from build123d import *

# Parameters (mm, degrees)
F0_R     = 2
F0_W     = 2.6
F0_H     = 107.6
F0_W_2   = 1.2
F0_H_2   = 1.2
F1_DEPTH = 1
F2_DEPTH = 10


with BuildPart() as f1:
    # F0 (on Top) → F1 (new body)
    with BuildSketch(Plane.XY):
        with BuildLine():
            ThreePointArc((65, 39.2), (57.4433549546, 57.4433549546), (39.2, 65))
            Line((39.2, 65), (-39.2, 65))
            ThreePointArc((-39.2, 65), (-57.4433549546, 57.4433549546), (-65, 39.2))
            Line((-65, 39.2), (-65, -39.2))
            ThreePointArc((-65, -39.2), (-57.4433549546, -57.4433549546), (-39.2, -65))
            Line((-39.2, -65), (39.2, -65))
            ThreePointArc((39.2, -65), (57.4433549546, -57.4433549546), (65, -39.2))
            Line((65, -39.2), (65, 39.2))
        make_face()
        with BuildLine():
            ThreePointArc((-58, -46.1086357947), (-61.4142135624, -47.5228493571), (-60, -44.1086357947))
            ThreePointArc((-60, -44.1086357947), (-58.5857864376, -44.6944222324), (-58, -46.1086357947))
        make_face(mode=Mode.SUBTRACT)
        with BuildLine():
            ThreePointArc((62, -46.1086357947), (58.5857864376, -47.5228493571), (60, -44.1086357947))
            ThreePointArc((60, -44.1086357947), (61.4142135624, -44.6944222324), (62, -46.1086357947))
        make_face(mode=Mode.SUBTRACT)
        with BuildLine():
            ThreePointArc((-58, 32.2913642053), (-58.5857864376, 30.8771506429), (-60, 30.2913642053))
            ThreePointArc((-60, 30.2913642053), (-61.4142135624, 33.7055777676), (-58, 32.2913642053))
        make_face(mode=Mode.SUBTRACT)
        with Locations((-39.2, 60)):
            Circle(F0_R, mode=Mode.SUBTRACT)
        with BuildLine():
            ThreePointArc((-55, 39.2), (-50.3722871427, 50.3722871427), (-39.2, 55))
            Line((-39.2, 55), (-2.5, 55))
            Line((-2.5, 55), (-1.3, 55))
            Line((-1.3, 55), (1.3, 55))
            Line((1.3, 55), (2.5, 55))
            Line((2.5, 55), (39.2, 55))
            ThreePointArc((39.2, 55), (50.3722871427, 50.3722871427), (55, 39.2))
            Line((55, 39.2), (55, -39.2))
            ThreePointArc((55, -39.2), (50.3722871427, -50.3722871427), (39.2, -55))
            Line((39.2, -55), (2.5, -55))
            Line((2.5, -55), (1.3, -55))
            Line((1.3, -55), (-1.3, -55))
            Line((-1.3, -55), (-2.5, -55))
            Line((-2.5, -55), (-39.2, -55))
            ThreePointArc((-39.2, -55), (-50.3722871427, -50.3722871427), (-55, -39.2))
            Line((-55, -39.2), (-55, 39.2))
        make_face(mode=Mode.SUBTRACT)
        with BuildLine():
            ThreePointArc((62, 32.2913642053), (61.4142135624, 30.8771506429), (60, 30.2913642053))
            ThreePointArc((60, 30.2913642053), (58.5857864376, 33.7055777676), (62, 32.2913642053))
        make_face(mode=Mode.SUBTRACT)
        with BuildLine():
            ThreePointArc((41.2, 60), (39.2, 58), (37.2, 60))
            ThreePointArc((37.2, 60), (39.2, 62), (41.2, 60))
        make_face(mode=Mode.SUBTRACT)
        Rectangle(F0_W, F0_H)
        with BuildLine():
            Line((-2.5, 55), (-39.2, 55))
            ThreePointArc((-39.2, 55), (-50.3722871427, 50.3722871427), (-55, 39.2))
            Line((-55, 39.2), (-55, -39.2))
            ThreePointArc((-55, -39.2), (-50.3722871427, -50.3722871427), (-39.2, -55))
            Line((-39.2, -55), (-2.5, -55))
            Line((-2.5, -55), (-2.5, -53.8))
            Line((-2.5, -53.8), (-38.8, -53.8))
            ThreePointArc((-38.8, -53.8), (-49.4066017178, -49.4066017178), (-53.8, -38.8))
            Line((-53.8, -38.8), (-53.8, 38.8))
            ThreePointArc((-53.8, 38.8), (-49.4066017178, 49.4066017178), (-38.8, 53.8))
            Line((-38.8, 53.8), (-2.5, 53.8))
            Line((-2.5, 53.8), (-2.5, 55))
        make_face()
        with BuildLine():
            Line((39.2, 55), (2.5, 55))
            Line((2.5, 55), (2.5, 53.8))
            Line((2.5, 53.8), (38.8, 53.8))
            ThreePointArc((38.8, 53.8), (49.4066017178, 49.4066017178), (53.8, 38.8))
            Line((53.8, 38.8), (53.8, -38.8))
            ThreePointArc((53.8, -38.8), (49.4066017178, -49.4066017178), (38.8, -53.8))
            Line((38.8, -53.8), (2.5, -53.8))
            Line((2.5, -53.8), (2.5, -55))
            Line((2.5, -55), (39.2, -55))
            ThreePointArc((39.2, -55), (50.3722871427, -50.3722871427), (55, -39.2))
            Line((55, -39.2), (55, 39.2))
            ThreePointArc((55, 39.2), (50.3722871427, 50.3722871427), (39.2, 55))
        make_face()
        with Locations((-1.9, 0)):
            Rectangle(F0_W_2, F0_H)
        with Locations((1.9, 0)):
            Rectangle(F0_W_2, F0_H)
        with BuildLine():
            ThreePointArc((-58, -46.1086357947), (-58.5857864376, -44.6944222324), (-60, -44.1086357947))
            ThreePointArc((-60, -44.1086357947), (-61.4142135624, -47.5228493571), (-58, -46.1086357947))
        make_face()
        with BuildLine():
            ThreePointArc((-58, 32.2913642053), (-61.4142135624, 33.7055777676), (-60, 30.2913642053))
            ThreePointArc((-60, 30.2913642053), (-58.5857864376, 30.8771506429), (-58, 32.2913642053))
        make_face()
        with Locations((-39.2, 60)):
            Circle(F0_R)
        with BuildLine():
            ThreePointArc((41.2, 60), (39.2, 62), (37.2, 60))
            ThreePointArc((37.2, 60), (39.2, 58), (41.2, 60))
        make_face()
        with BuildLine():
            ThreePointArc((62, 32.2913642053), (58.5857864376, 33.7055777676), (60, 30.2913642053))
            ThreePointArc((60, 30.2913642053), (61.4142135624, 30.8771506429), (62, 32.2913642053))
        make_face()
        with BuildLine():
            ThreePointArc((62, -46.1086357947), (61.4142135624, -44.6944222324), (60, -44.1086357947))
            ThreePointArc((60, -44.1086357947), (58.5857864376, -47.5228493571), (62, -46.1086357947))
        make_face()
        with Locations((0, -54.4)):
            Rectangle(F0_W, F0_H_2)
        with Locations((0, 54.4)):
            Rectangle(F0_W, F0_H_2)
        with Locations((-1.9, -54.4)):
            Rectangle(F0_W_2, F0_H_2)
        with Locations((1.9, -54.4)):
            Rectangle(F0_W_2, F0_H_2)
        with Locations((-1.9, 54.4)):
            Rectangle(F0_W_2, F0_H_2)
        with Locations((1.9, 54.4)):
            Rectangle(F0_W_2, F0_H_2)
    extrude(amount=F1_DEPTH)

    # F0 (on Top) → F2 (join)
    with BuildSketch(Plane.XY):
        with BuildLine():
            ThreePointArc((-58, -46.1086357947), (-58.5857864376, -44.6944222324), (-60, -44.1086357947))
            ThreePointArc((-60, -44.1086357947), (-61.4142135624, -47.5228493571), (-58, -46.1086357947))
        make_face()
        with BuildLine():
            ThreePointArc((-58, 32.2913642053), (-61.4142135624, 33.7055777676), (-60, 30.2913642053))
            ThreePointArc((-60, 30.2913642053), (-58.5857864376, 30.8771506429), (-58, 32.2913642053))
        make_face()
        with BuildLine():
            ThreePointArc((41.2, 60), (39.2, 62), (37.2, 60))
            ThreePointArc((37.2, 60), (39.2, 58), (41.2, 60))
        make_face()
        with Locations((-39.2, 60)):
            Circle(F0_R)
        with BuildLine():
            ThreePointArc((62, -46.1086357947), (61.4142135624, -44.6944222324), (60, -44.1086357947))
            ThreePointArc((60, -44.1086357947), (58.5857864376, -47.5228493571), (62, -46.1086357947))
        make_face()
        with BuildLine():
            ThreePointArc((62, 32.2913642053), (58.5857864376, 33.7055777676), (60, 30.2913642053))
            ThreePointArc((60, 30.2913642053), (61.4142135624, 30.8771506429), (62, 32.2913642053))
        make_face()
    extrude(amount=F2_DEPTH)


solid = f1.part
For this review, take the finished solid that the model builds, in its own axes (mm). A direction names the side the tool comes from. Round coordinates to 2 decimals unless told otherwise and drop trailing zeros. Write each loop counter-clockwise with the first axis right and the second up, starting at its lowest first coordinate (ties: lowest second). Pieces come first, ordered by that corner, then holes. Notation, with made-up numbers: (-9, 54.5) - (48, 54.5) arc R20 cw to (48, 87.5) - close; hole circle Ø8 at (8, 43.5). An arc over 180 degrees is marked (long way). Write item = value, one per line. Start each with the question number.
1. Wall thickness on L1, parallel to X at y = -11, z = 0.5; L2, parallel to Y at x = 58.5, z = 6.25; L3, parallel to Z at x = 49.5, y = 54: over which ranges is each line inside the solid? List them lowest first.
2. Consider section D-D on y = 44. State the section outline as (x, z) points, plus the area to 3 significant figures.
3. Consider section B-B on y = -13.5. State the section outline as (x, z) points.
4. Consider section A-A on x = 14.5. State the section outline as (y, z) points.
5. For pin 1 Ø3 at (x, z) = (-40.5, 2) entering from +Y, flat-tipped, find the tip position at first contact; note if it passes through.
6. Draft analysis for pull direction X (two halves, no side actions). For faces 4 (the face through (57.242, -57.643, 0.493)), 5 (the face through (-60, 32, 10)), 6 (the face through (-49.29, -49.52, 0.49)), 7 (the face through (49.29, 49.52, 0.49)), state which applies: released by +X, released by -X, zero draft, split by the parting line, or undercut.
7. Consider section C-C on z = 2.5. State the section outline as (x, y) points.
8. For faces 1 (the face through (49.52, -49.29, 0.49)), 2 (the face through (60, 32, 10)), 3 (the face through (-38.125, 61.686, 5.437)), list the 3-axis set-ups (+Z, -Z, +X, -X, +Y, -Y) from which the entire face can be reached by the end or side of a thin tool; tool diameter is ignored.
Evaluation:
q1.L1 = -65 to -53.8, -2.5 to 2.5, 53.8 to 65
q1.L2 = -47.43 to -44.79, 30.97 to 33.61
q1.L3 = 0 to 1
q2.outline = (-64.55, 0) - (-52.87, 0) - (-52.87, 1) - (-64.55, 1) - close; (-2.5, 0) - (2.5, 0) - (2.5, 1) - (-2.5, 1) - close; (52.87, 0) - (64.55, 0) - (64.55, 1) - (52.87, 1) - close
q2.area = 28.4 mm2
q3.outline = (-65, 0) - (-53.8, 0) - (-53.8, 1) - (-65, 1) - close; (-2.5, 0) - (2.5, 0) - (2.5, 1) - (-2.5, 1) - close; (53.8, 0) - (65, 0) - (65, 1) - (53.8, 1) - close
q4.outline = (-65, 0) - (-53.8, 0) - (-53.8, 1) - (-65, 1) - close; (53.8, 0) - (65, 0) - (65, 1) - (53.8, 1) - close
q5.pin_1 = 65
q6.face_4 = released by +X
q6.face_5 = zero draft
q6.face_6 = undercut
q6.face_7 = undercut
q7.outline = circle Ø4 at (-60, -46.11); circle Ø4 at (-60, 32.29); circle Ø4 at (-39.2, 60); circle Ø4 at (39.2, 60); circle Ø4 at (60, -46.11); circle Ø4 at (60, 32.29)
q8.face_1 = +Z, -Z
q8.face_2 = +Z, +X, -X, +Y, -Y
q8.face_3 = +Z
